Read the model definition and answer for the solid it produces. Units are mm, in the model's axes. Face numbers are marked on the shaded views. A direction names the side the tool comes from. Coordinates: 2 decimals unless noted, no trailing zeros. Loops run counter-clockwise (first coordinate to the right, second up) from the corner with the lowest first, then second, coordinate; pieces in that order, holes last.
from build123d import *

# Parameters (mm, degrees)
BOSS_EXTRUDE1_DEPTH = 5
SKETCH3_W           = 8
SKETCH3_H           = 4
BOSS_EXTRUDE2_DEPTH = 3
FILLET1_START       = -3.841593316
FILLET1_DEPTH       = 8
CUT_EXTRUDE1_START  = -10
CUT_EXTRUDE1_DEPTH  = 10
FILLET2_R           = 3
SKETCH6_R           = 1.5
CUT_EXTRUDE2_DEPTH  = 5
SKETCH7_R           = 1.25
CUT_EXTRUDE3_DEPTH  = 5


with BuildPart() as part:
    # Sketch1 → Boss-Extrude1 (new body)
    with BuildSketch(Plane(origin=(0, 0, 0), x_dir=(1, 0, 0), z_dir=(0, 1, 0))):
        with BuildLine():
            Line((-30, 0), (30, 0))
            ThreePointArc((30, 0), (0, 30), (-30, 0))
        make_face()
    extrude(amount=BOSS_EXTRUDE1_DEPTH)

    # Sketch3 → Boss-Extrude2 (add)
    with BuildSketch(Plane(origin=(0, 5, 0), x_dir=(1, 0, 0), z_dir=(0, 1, 0))):
        with Locations((0.158406684, 24.731666579)):
            Rectangle(SKETCH3_W, SKETCH3_H)
    extrude(amount=BOSS_EXTRUDE2_DEPTH)

    # Fillet1: read off the stored shape, not the designer's step
    # Fillet1 outline → Fillet1 (cut)
    with BuildSketch(Plane.YZ.offset(FILLET1_START)):
        with BuildLine():
            Line((8, -22.731666579), (5, -22.731666579))
            add(Edge.make_bspline(
                [(5, -22.731666579), (8, -23.506263249), (8, -26.604649926)],
                knots=[0, 0, 0, 1, 1, 1], degree=2, weights=[1, 0.057495957, 1]))
            Line((8, -26.604649926), (8, -22.731666579))
        make_face()
    extrude(amount=FILLET1_DEPTH, mode=Mode.SUBTRACT)

    # Sketch5 → Cut-Extrude1 (cut)
    with BuildSketch(Plane(origin=(0, 5, 0), x_dir=(1, 0, 0), z_dir=(0, 1, 0)).offset(CUT_EXTRUDE1_START)):
        with BuildLine():
            Line((-21.393876913, 0), (-21.393876913, 6))
            Line((-21.393876913, 6), (-29.393876913, 6))
            ThreePointArc((-29.393876913, 6), (-29.84808459, 3.01526886), (-30, 0))
            Line((-30, 0), (-21.393876913, 0))
        make_face()
        with BuildLine():
            Line((21.393876913, 6), (29.393876913, 6))
            ThreePointArc((29.393876913, 6), (29.84808459, 3.01526886), (30, 0))
            Line((30, 0), (21.393876913, 0))
            Line((21.393876913, 0), (21.393876913, 6))
        make_face()
    extrude(amount=CUT_EXTRUDE1_DEPTH, mode=Mode.SUBTRACT)

    # Fillet2
    fillet2_edges = [part.edges().sort_by_distance(p)[0] for p in [
        (0, 5, 0),
    ]]
    fillet(fillet2_edges, radius=FILLET2_R)

    # Sketch6 → Cut-Extrude2 (cut)
    with BuildSketch(Plane(origin=(21.393876913, 0, 0), x_dir=(0, 0, -1), z_dir=(1, 0, 0))):
        with Locations((3, 2.25)):
            Circle(SKETCH6_R)
    extrude(amount=-CUT_EXTRUDE2_DEPTH, mode=Mode.SUBTRACT)

    # Sketch7 → Cut-Extrude3 (cut)
    with BuildSketch(Plane.ZY.offset(21.393876913)):
        with Locations((-3, 2.25)):
            Circle(SKETCH7_R)
    extrude(amount=-CUT_EXTRUDE3_DEPTH, mode=Mode.SUBTRACT)


solid = part.part
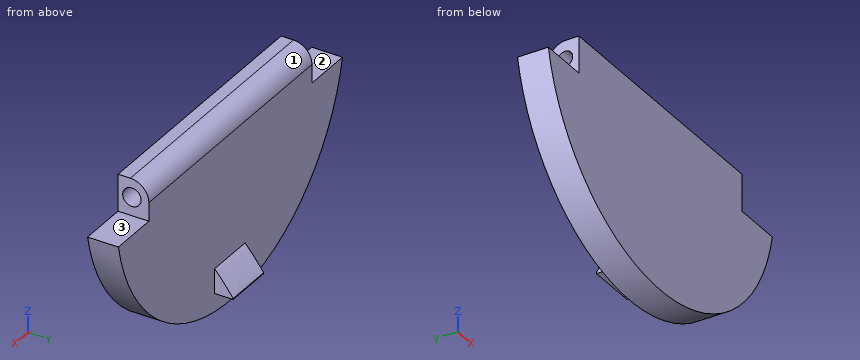
Item 1: A cutting plane is placed at D-D on z = -15. Determine the outline of the cut face in (x, y).
Numbers:
outline: (-25.98, 0) - (25.98, 0) - (25.98, 5) - (-25.98, 5) - close
Item 2: A cutting plane is placed at A-A on x = -18.5. Determine the outline of the cut face in (y, z), then the cut area to 3 significant figures.
Numbers:
outline: (0, -23.62) - (5, -23.62) - (5, -3) arc R3 ccw to (2, 0) - (0, 0) - close; hole circle Ø2.5 at (2.25, -3)
area: 111 mm2
Item 3: Find the intervals of material crossed by line 1 along X through (y, z) = (3.5, -4.5); line 2 along Y through (x, z) = (-17, -21); line 3 along Z through (x, y) = (-19.5, 3), in increasing order.
Numbers:
line 1: x = -21.39 to 21.39
line 2: y = 0 to 5
line 3: z = -22.8 to -4, -2 to -0.17
Item 4: Which of the six approach directions +Z, -Z, +X, -X, +Y, -Y give full straight-line access (tool end or side, diameter ignored) to the marked faces 1, 2 and 3?
Numbers:
face 1: +Z, +X, -X, +Y
face 2: +Z, -X, +Y, -Y
face 3: +Z, +X, +Y, -Y
Item 5: Given pin 1 (2.5 mm diameter, centred on x = 2, y = 7, fed in from -Z); pin 2 (8 mm diameter, centred on x = 7.5, z = -17, fed in from +Y); pin 3 (2 mm diameter, centred on y = 2.25, z = -3, fed in from -X), each flat-ended and moving along its own axis, determine where each tip first touches the part or whether it passes through.
Numbers:
pin 1: stops at z = -26.73
pin 2: stops at y = 5
pin 3: stops at x = -16.39
Item 6: A cutting plane is placed at B-B on x = 15.5. Determine the outline of the cut face in (y, z), then the cut area to 3 significant figures.
Numbers:
outline: (0, -25.69) - (5, -25.69) - (5, -3) arc R3 ccw to (2, 0) - (0, 0) - close
area: 126 mm2
Item 7: A cutting plane is placed at C-C on z = -20. Determine the outline of the cut face in (x, y), then the cut area to 3 significant figures.
Numbers:
outline: (-22.36, 0) - (22.36, 0) - (22.36, 5) - (-22.36, 5) - close
area: 224 mm2
